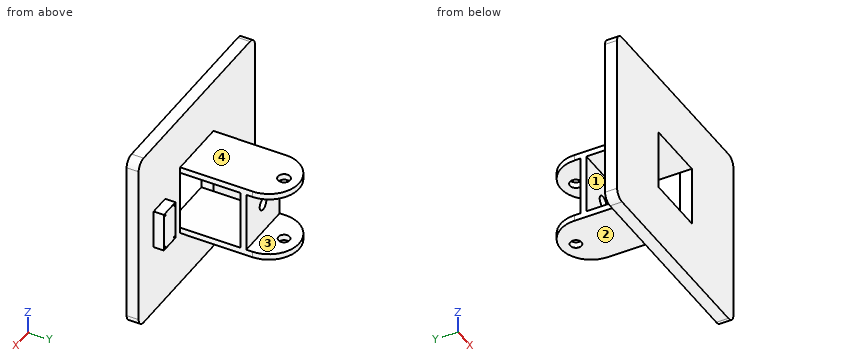
```python
from build123d import *

# Parameters (mm, degrees)
SKETCH1_W                              = 350
SKETCH1_H                              = 300
BOSS_EXTRUDE1_DEPTH                    = 20
FILLET1_R                              = 15
SKETCH2_W                              = 100
SKETCH2_H                              = 100
CUT_EXTRUDE1_DEPTH                     = 20
BOSS_EXTRUDE2_DEPTH                    = 10
LPATTERN1_COUNT                        = 2
LPATTERN1_PITCH                        = 110
F_20_0_20_DIAMETER_HOLE2_D             = 20
F_20_0_20_DIAMETER_HOLE2_DEPTH         = 10
F_20_0_20_DIAMETER_HOLE2_CSINK_D       = 20.05
F_20_0_20_DIAMETER_HOLE2_CSINK_ANGLE   = 90
F_20_0_20_DIAMETER_HOLE2_TIP           = 6.00860619
F_18_5_18_5_DIAMETER_HOLE1_D           = 18.5
F_18_5_18_5_DIAMETER_HOLE1_DEPTH       = 10
F_18_5_18_5_DIAMETER_HOLE1_CSINK_D     = 18.55
F_18_5_18_5_DIAMETER_HOLE1_CSINK_ANGLE = 90
F_18_5_18_5_DIAMETER_HOLE1_TIP         = 5.557960726
SKETCH32_W                             = 100
SKETCH32_H                             = 10
BOSS_EXTRUDE3_DEPTH                    = 120
SKETCH37_R                             = 10
CUT_EXTRUDE2_DEPTH                     = 36.07831716
SKETCH45_W                             = 35
SKETCH45_H                             = 65
BOSS_EXTRUDE4_DEPTH                    = 17
M2_5_CLEARANCE_HOLE1_D                 = 2.9
M2_5_CLEARANCE_HOLE1_DEPTH             = 12.4
M2_5_CLEARANCE_HOLE1_CSINK_D           = 2.95
M2_5_CLEARANCE_HOLE1_CSINK_ANGLE       = 90
M2_5_CLEARANCE_HOLE1_TIP               = 0.871247898


with BuildPart() as part:
    # Sketch1 → Boss-Extrude1 (new body)
    with BuildSketch(Plane(origin=(0, 0, 0), x_dir=(1, 0, 0), z_dir=(0, 1, 0))):
        with Locations((175, -150)):
            Rectangle(SKETCH1_W, SKETCH1_H)
    extrude(amount=BOSS_EXTRUDE1_DEPTH)

    # Fillet1
    fillet1_edges = [part.edges().sort_by_distance(p)[0] for p in [
        (0, 10, 0),
        (350, 10, 0),
        (350, 10, 300),
        (0, 10, 300),
    ]]
    fillet(fillet1_edges, radius=FILLET1_R)

    # Sketch2 → Cut-Extrude1 (cut)
    with BuildSketch(Plane(origin=(0, 20, 0), x_dir=(1, 0, 0), z_dir=(0, 1, 0))):
        with Locations((175, -150)):
            Rectangle(SKETCH2_W, SKETCH2_H)
    extrude(amount=-CUT_EXTRUDE1_DEPTH, mode=Mode.SUBTRACT)

    # Sketch6 → Boss-Extrude2 (add)
    with BuildSketch(Plane.XY.offset(100)):
        with BuildLine():
            Line((125, 0), (125, 140))
            ThreePointArc((125, 140), (175, 190), (225, 140))
            Line((225, 140), (225, 0))
            Line((225, 0), (125, 0))
        make_face()
    boss_extrude2 = extrude(amount=-BOSS_EXTRUDE2_DEPTH)

    # LPattern1: Boss-Extrude2 ×2
    with Locations(*[(0, 0, i * LPATTERN1_PITCH) for i in range(1, LPATTERN1_COUNT)]):
        add(boss_extrude2)

    # Ø20.0 (20) Diameter Hole2
    with Locations(Plane.XY.offset(210)):
        with Locations((175, 165)):
            CounterSinkHole(F_20_0_20_DIAMETER_HOLE2_D / 2, F_20_0_20_DIAMETER_HOLE2_CSINK_D / 2, depth=F_20_0_20_DIAMETER_HOLE2_DEPTH, counter_sink_angle=F_20_0_20_DIAMETER_HOLE2_CSINK_ANGLE)
            with Locations((0, 0, -(F_20_0_20_DIAMETER_HOLE2_DEPTH + F_20_0_20_DIAMETER_HOLE2_TIP / 2))):  # 118° drill point
                Cone(0, F_20_0_20_DIAMETER_HOLE2_D / 2, F_20_0_20_DIAMETER_HOLE2_TIP, mode=Mode.SUBTRACT)

    # Ø18.5 (18.5) Diameter Hole1
    with Locations(Plane(origin=(0, 0, 90), x_dir=(-1, 0, 0), z_dir=(0, 0, -1))):
        with Locations((-175, 165)):
            CounterSinkHole(F_18_5_18_5_DIAMETER_HOLE1_D / 2, F_18_5_18_5_DIAMETER_HOLE1_CSINK_D / 2, depth=F_18_5_18_5_DIAMETER_HOLE1_DEPTH, counter_sink_angle=F_18_5_18_5_DIAMETER_HOLE1_CSINK_ANGLE)
            with Locations((0, 0, -(F_18_5_18_5_DIAMETER_HOLE1_DEPTH + F_18_5_18_5_DIAMETER_HOLE1_TIP / 2))):  # 118° drill point
                Cone(0, F_18_5_18_5_DIAMETER_HOLE1_D / 2, F_18_5_18_5_DIAMETER_HOLE1_TIP, mode=Mode.SUBTRACT)

    # Sketch32 → Boss-Extrude3 (add)
    with BuildSketch(Plane.XY.offset(210)):
        with Locations((175, 125)):
            Rectangle(SKETCH32_W, SKETCH32_H)
    extrude(amount=-BOSS_EXTRUDE3_DEPTH)

    # Sketch37 → Cut-Extrude2 (cut)
    with BuildSketch(Plane(origin=(0, 130, 0), x_dir=(1, 0, 0), z_dir=(0, 1, 0))):
        with Locations((175, -150)):
            Circle(SKETCH37_R)
    extrude(amount=-CUT_EXTRUDE2_DEPTH, mode=Mode.SUBTRACT)

    # Sketch45 → Boss-Extrude4 (add)
    with BuildSketch(Plane(origin=(0, 20, 0), x_dir=(1, 0, 0), z_dir=(0, 1, 0))):
        with Locations((287.5, -150)):
            Rectangle(SKETCH45_W, SKETCH45_H)
    extrude(amount=BOSS_EXTRUDE4_DEPTH)

    # M2.5 Clearance Hole1
    with Locations(Plane(origin=(0, 37, 0), x_dir=(1, 0, 0), z_dir=(0, 1, 0))):
        with Locations((273.5, -121), (301.5, -121), (301.5, -179), (273.5, -179)):
            CounterSinkHole(M2_5_CLEARANCE_HOLE1_D / 2, M2_5_CLEARANCE_HOLE1_CSINK_D / 2, depth=M2_5_CLEARANCE_HOLE1_DEPTH, counter_sink_angle=M2_5_CLEARANCE_HOLE1_CSINK_ANGLE)
            with Locations((0, 0, -(M2_5_CLEARANCE_HOLE1_DEPTH + M2_5_CLEARANCE_HOLE1_TIP / 2))):  # 118° drill point
                Cone(0, M2_5_CLEARANCE_HOLE1_D / 2, M2_5_CLEARANCE_HOLE1_TIP, mode=Mode.SUBTRACT)


solid = part.part
```
The listing builds one solid part. Answer for the finished solid, in the listing's coordinates (mm). Face numbers are marked on the shaded views. A direction names the side the tool comes from. Round coordinates to 2 decimals unless told otherwise and drop trailing zeros. Write each loop counter-clockwise with the first axis right and the second up, starting at its lowest first coordinate (ties: lowest second). Pieces come first, ordered by that corner, then holes. Notation, with made-up numbers: (32.5, 14) -> (65.5, 14) arc R14 cw to (65.5, 31) -> close; hole circle Ø5 at (-9.75, -1). An arc over 180 degrees is marked (long way). Answer as a JSON object with one key per item and string values. Group by question number.
Q1. Section A-A (z = 150) is taken. Write down the section's boundary in (x, y).
Q2. Straight lines are drawn through the part: line 1 along Z through (x, y) = (301, 29); line 2 along Z through (x, y) = (220, 76.5); line 3 along Y through (x, z) = (175, 97). For each, find the intervals that lie inside material, in ascending order.
Q3. Section C-C (x = 175) is taken. Count the separate pieces of the cut face and the enclosed holes in it, plus the area to 4 significant figures.
Q4. Section D-D (y = 165) is taken. Write down the section's boundary in (x, z) (3 decimals), plus the area to 3 significant figures.
Q5. Each of these flat-tipped pins is pushed along its axis until it touches: pin 1 Ø3.5 at (x, z) = (273.5, 179) entering from +Y; pin 2 Ø5 at (x, z) = (256.5, 101.5) entering from +Y; pin 3 Ø8.5 at (y, z) = (30.5, 139) entering from -X; pin 4 Ø1.7 at (x, z) = (301.5, 121) entering from -Y. Where does it stop, or does it pass through?
Q6. Section B-B (y = 97.5) is taken. Write down the section's boundary in (x, z), plus the area to 3 significant figures.
Q7. Which of the six approach directions +Z, -Z, +X, -X, +Y, -Y give full straight-line access (tool end or side, diameter ignored) to the marked faces 1, 2, 3 and 4?
Check values:
{
 "1": {"outline": "(0, 0) -> (125, 0) -> (125, 20) -> (0, 20) -> close; (125, 120) -> (165, 120) -> (165, 130) -> (125, 130) -> close; (185, 120) -> (225, 120) -> (225, 130) -> (185, 130) -> close; (225, 0) -> (350, 0) -> (350, 20) -> (305, 20) -> (305, 37) -> (270, 37) -> (270, 20) -> (225, 20) -> close"},
 "2": {"line 1": "117.5 to 119.64, 122.36 to 177.64, 180.36 to 182.5", "line 2": "90 to 100, 200 to 210", "line 3": "0 to 155.75, 174.25 to 190"},
 "3": {"separate pieces": "4", "enclosed holes": "0", "area": "7,815 mm^2"},
 "4": {"outline": "(131.699, 90) -> (165.725, 90) -> (165.75, 90.025) -> (165.75, 100) -> (131.699, 100) -> close; (131.699, 200) -> (165, 200) -> (165, 209.975) -> (164.975, 210) -> (131.699, 210) -> close; (184.25, 90.025) -> (184.275, 90) -> (218.301, 90) -> (218.301, 100) -> (184.25, 100) -> close; (185, 200) -> (218.301, 200) -> (218.301, 210) -> (185.025, 210) -> (185, 209.975) -> close", "area": "1,350 mm^2"},
 "5": {"pin 1": "y = 37", "pin 2": "y = 20", "pin 3": "x = 270", "pin 4": "y = 0"},
 "6": {"outline": "(125, 90) -> (225, 90) -> (225, 100) -> (125, 100) -> close; (125, 200) -> (225, 200) -> (225, 210) -> (125, 210) -> close", "area": "2,000 mm^2"},
 "7": {"face 1": "+X, -X, -Y", "face 2": "-Z, +X, -X, +Y", "face 3": "+X, -X, +Y", "face 4": "+Z, +X, -X, +Y"}
}
